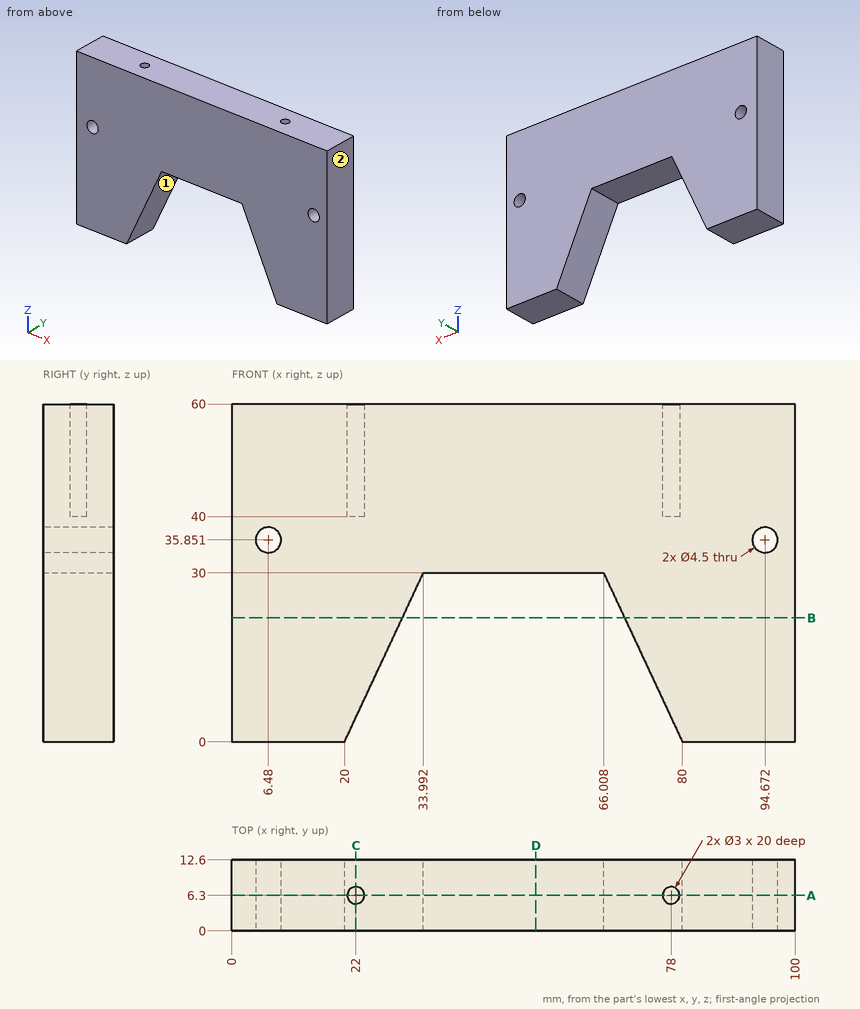
Answer from the drawing. Dimensions are ordinates in mm from the lowest x, y and z of the part. A direction names the side the tool comes from. Give positions to 0.01 mm unless a question says otherwise; leave off trailing zeros. Order: outer loops, then holes, each group sorted by start corner. A loop starts at its lowest first (then second) coordinate and runs counter-clockwise, first axis right, second up. Notation, with made-up numbers: (-7.5, 80.5) -> (27.5, 80.5) arc R18 ccw to (27.5, 114.5) -> close; hole circle Ø2 at (79.25, -14). An arc over 180 degrees is marked (long way). Answer as a JSON object with one key per item and string values. Group by question number.
1. Consider line 1 along Y through (x, z) = (78, 50.5); line 2 along Z through (x, y) = (41, 11.5); line 3 along X through (y, z) = (11.5, 17). Determine where each line is inside the solid, lowest interval first. Write a range as [from, to].
2. Section B-B on z = 22 is taken. Determine the outline of the cut face in (x, y).
3. Section A-A on y = 6.3 is taken. Determine the outline of the cut face in (x, z), plus the area to 3 significant figures.
4. A tool of negligible diameter and unlimited length cuts with its end or side. For the marked faces 1 and 2, from which of +Z, -Z, +X, -X, +Y, -Y can it reach the whole face along a straight path? Write none if from no direction.
5. Section C-C on x = 22 is taken. Determine the outline of the cut face in (y, z), plus the area to 3 significant figures.
6. Flat-ended cylindrical pins translate along their axes: pin 1 Ø0.9 at (x, y) = (78.5, 6) entering from +Z; pin 2 Ø4 at (x, y) = (23.5, 4.5) entering from -Z (1 decimal); pin 3 Ø2.5 at (x, y) = (78, 6.3) entering from -Z. Find the tip coordinate at first contact, or state that the pin passes through.
7. Section D-D on x = 54 is taken. Determine the outline of the cut face in (y, z).
Result sheet:
{
 "1": {"line 1": "y = [0, 4.8], [7.8, 12.6]", "line 2": "z = [30, 60]", "line 3": "x = [0, 27.93], [72.07, 100]"},
 "2": {"outline": "(0, 0) -> (30.26, 0) -> (30.26, 12.6) -> (0, 12.6) -> close; (69.74, 0) -> (100, 0) -> (100, 12.6) -> (69.74, 12.6) -> close"},
 "3": {"outline": "(0, 0) -> (20, 0) -> (33.99, 30) -> (66.01, 30) -> (80, 0) -> (100, 0) -> (100, 60) -> (79.5, 60) -> (79.5, 40) -> (76.5, 40) -> (76.5, 60) -> (23.5, 60) -> (23.5, 40) -> (20.5, 40) -> (20.5, 60) -> (0, 60) -> close; hole circle Ø4.5 at (6.48, 35.85); hole circle Ø4.5 at (94.67, 35.85)", "area": "4,470 mm^2"},
 "4": {"face 1": "-Z, +Y, -Y", "face 2": "+Z, -Z, +X, +Y, -Y"},
 "5": {"outline": "(0, 4.29) -> (12.6, 4.29) -> (12.6, 60) -> (7.8, 60) -> (7.8, 40) -> (4.8, 40) -> (4.8, 60) -> (0, 60) -> close", "area": "642 mm^2"},
 "6": {"pin 1": "stops at z = 40", "pin 2": "stops at z = 3.2", "pin 3": "stops at z = 1.61"},
 "7": {"outline": "(0, 30) -> (12.6, 30) -> (12.6, 60) -> (0, 60) -> close"}
}
